Could you check a few things on this model? Use its own coordinates, in mm. A direction names the side the tool comes from. Coordinates: 2 decimals unless noted, no trailing zeros. Write each loop counter-clockwise with the first axis right and the second up, starting at its lowest first coordinate (ties: lowest second). Pieces come first, ordered by that corner, then holes. Notation, with made-up numbers: (-15.75, 87) - (40.25, 87) arc R16 cw to (40.25, 106) - close; hole circle Ø5 at (51, 68.5). An arc over 180 degrees is marked (long way). Answer as a JSON object with one key per item and string values. Group by question number.
1) On a 3-axis mill with a long thin cutter (end or side, diameter ignored), from which of +Z, -Z, +X, -X, +Y, -Y can I reach the whole of each face in a straight line? I mean faces 1 (the flat face through (10, 13, 3)), 2 (the flat face through (0, 0, 3)). Say none if no direction works.
2) If we section it at B-B (x = 4.75): Write out the boundary of the cut face in (y, z).
3) Will these pins go through, and if not, where does the flat tip stop? pin 1 Ø1.9 at (x, y) = (4.75, 16) entering from +Z; pin 2 Ø3 at (y, z) = (12, 5.5) entering from +X.
4) If we section it at A-A (z = 3.5): Write out the boundary of the cut face in (x, y) (3 decimals), plus the area to 3 significant figures.
5) If we section it at D-D (y = 16): Write out the boundary of the cut face in (x, z), plus the area to 3 significant figures.
6) If we section it at C-C (y = 1.5): Write out the boundary of the cut face in (x, z) (3 decimals).
7) Please list where these lines run through material, in increasing order: line 1 along Y through (x, z) = (4.75, 1.5); line 2 along Z through (x, y) = (13.5, 2.8) (3 decimals); line 3 along X through (y, z) = (19, 5).
8) We'd pull the mould along X, two halves only. Please class faces 3 (the cylindrical face through (-13.434, 2.535, 5.174)), 4 (the cylindrical face through (13.566, 2.535, 5.174)), 5 (the flat face through (-10, 14, 3)), 6 (the flat face through (0, 22, 3)): released by +X, released by -X, zero draft, split by the parting line, or undercut.
```python
from build123d import *

# Parameters (mm, degrees)
SKETCH2_R           = 1.05
BOSS_EXTRUDE1_DEPTH = 7
CUT_EXTRUDE1_DEPTH  = 26.039968051


with BuildPart() as part:
    # Sketch2 → Boss-Extrude1 (new body)
    with BuildSketch(Plane.XY):
        Polygon((-10, 5), (-17, 5), (-17, 0), (17, 0), (17, 5), (10, 5), (10, 22), (-10, 22), align=None)
        with Locations((-4.75, 16)):
            Circle(SKETCH2_R, mode=Mode.SUBTRACT)
        with Locations(Location((4.75, 16, 0), (0, 0, 180))):
            Circle(SKETCH2_R, mode=Mode.SUBTRACT)
    extrude(amount=BOSS_EXTRUDE1_DEPTH)

    # Sketch3 → Cut-Extrude1 (cut, through all)
    with BuildSketch(Plane(origin=(0, 5, 0), x_dir=(1, 0, 0), z_dir=(0, 1, 0))):
        with BuildLine():
            Line((-13.5, -1.72667493), (-12.95, -1.917873267))
            ThreePointArc((-12.95, -1.917873267), (-13.5, -5.175), (-14.05, -1.917873267))
            Line((-14.05, -1.917873267), (-13.5, -1.72667493))
        make_face()
        with BuildLine():
            Line((13.5, -1.72667493), (14.05, -1.917873267))
            ThreePointArc((14.05, -1.917873267), (13.5, -5.175), (12.95, -1.917873267))
            Line((12.95, -1.917873267), (13.5, -1.72667493))
        make_face()
    extrude(amount=-CUT_EXTRUDE1_DEPTH, mode=Mode.SUBTRACT)


solid = part.part
```
Here are the results:
{
 "1": {"face 1": "+Z, -Z, +X, +Y", "face 2": "+Z, -Z, +X, -X, -Y"},
 "2": {"outline": "(0, 0) - (14.95, 0) - (14.95, 7) - (0, 7) - close; (17.05, 0) - (22, 0) - (22, 7) - (17.05, 7) - close"},
 "3": {"pin 1": "passes through", "pin 2": "stops at x = 10"},
 "4": {"outline": "(-17, 0) - (-15.175, 0) - (-15.175, 5) - (-17, 5) - close; (-11.825, 0) - (11.825, 0) - (11.825, 5) - (10, 5) - (10, 22) - (-10, 22) - (-10, 5) - (-11.825, 5) - close; (15.175, 0) - (17, 0) - (17, 5) - (15.175, 5) - close; hole circle Ø2.1 at (-4.75, 16); hole circle Ø2.1 at (4.75, 16)", "area": "470 mm²"},
 "5": {"outline": "(-10, 0) - (-5.8, 0) - (-5.8, 7) - (-10, 7) - close; (-3.7, 0) - (3.7, 0) - (3.7, 7) - (-3.7, 7) - close; (5.8, 0) - (10, 0) - (10, 7) - (5.8, 7) - close", "area": "111 mm²"},
 "6": {"outline": "(-17, 0) - (17, 0) - (17, 7) - (-17, 7) - close; hole (-14.05, 1.918) - (-13.5, 1.727) - (-12.95, 1.918) arc R1.675 ccw (long way) to start; hole (12.95, 1.918) - (13.5, 1.727) - (14.05, 1.918) arc R1.675 ccw (long way) to start"},
 "7": {"line 1": "y = 0 to 14.95, 17.05 to 22", "line 2": "z = 0 to 1.727, 5.175 to 7", "line 3": "x = -10 to 10"},
 "8": {"face 3": "undercut", "face 4": "undercut", "face 5": "released by -X", "face 6": "zero draft"}
}
